from build123d import *

# Parameters (mm, degrees)
SKETCH5_R           = 3.175
BOSS_EXTRUDE3_DEPTH = 88.9
CHAMFER1_SIZE       = 0.77724
BOSS_EXTRUDE4_DEPTH = 4.365625
SKETCH8_OUTSIDE_W   = 358.618
SKETCH8_OUTSIDE_H   = 360.338
SKETCH8_OUTSIDE_R   = 5.55625
CUT_EXTRUDE3_DEPTH  = 94.265625
CUT_EXTRUDE3_TAPER  = 60
CUT_EXTRUDE4_DEPTH  = 0.254
CIRPATTERN1_COUNT   = 3


with BuildPart() as part:
    # Sketch5 → Boss-Extrude3 (new body)
    with BuildSketch(Plane(origin=(46.6328125, 0, 0), x_dir=(0, 0, -1), z_dir=(1, 0, 0))):
        Circle(SKETCH5_R)
    extrude(amount=-BOSS_EXTRUDE3_DEPTH)

    # Chamfer1
    chamfer1_edges = [part.edges().sort_by_distance(p)[0] for p in [
        (46.6328125, 0, 3.175),
    ]]
    chamfer(chamfer1_edges, length=CHAMFER1_SIZE)

    # Sketch6 → Boss-Extrude4 (add)
    with BuildSketch(Plane.ZY.offset(42.2671875)):
        Polygon((5.55625, 3.207902433), (0, 6.415804866), (-5.55625, 3.207902433), (-5.55625, -3.207902433), (0, -6.415804866), (5.55625, -3.207902433), align=None)
    extrude(amount=BOSS_EXTRUDE4_DEPTH)

    # Sketch8 outside → Cut-Extrude3 (cut, through all)
    with BuildSketch(Plane.ZY.offset(46.6328125)):
        Rectangle(SKETCH8_OUTSIDE_W, SKETCH8_OUTSIDE_H)
        Circle(SKETCH8_OUTSIDE_R, mode=Mode.SUBTRACT)
    extrude(amount=-CUT_EXTRUDE3_DEPTH, taper=CUT_EXTRUDE3_TAPER, mode=Mode.SUBTRACT)

    # Sketch12 → Cut-Extrude4 (cut)
    with BuildSketch(Plane.ZY.offset(46.6328125)):
        with BuildLine():
            Line((0.1666875, 4.2783125), (0.1666875, 2.3891875))
            ThreePointArc((0.1666875, 2.3891875), (0, 2.2225), (-0.1666875, 2.3891875))
            Line((-0.1666875, 2.3891875), (-0.1666875, 4.2783125))
            ThreePointArc((-0.1666875, 4.2783125), (0, 4.445), (0.1666875, 4.2783125))
        make_face()
    cut_extrude4 = extrude(amount=-CUT_EXTRUDE4_DEPTH, mode=Mode.SUBTRACT)

    # CirPattern1: Cut-Extrude4 ×3 about axis
    cirpattern1_axis = Axis((0, 0, 0), (1, 0, 0))
    for i in range(1, CIRPATTERN1_COUNT):
        add(cut_extrude4.rotate(cirpattern1_axis, i * 360 / CIRPATTERN1_COUNT), mode=Mode.SUBTRACT)


solid = part.part
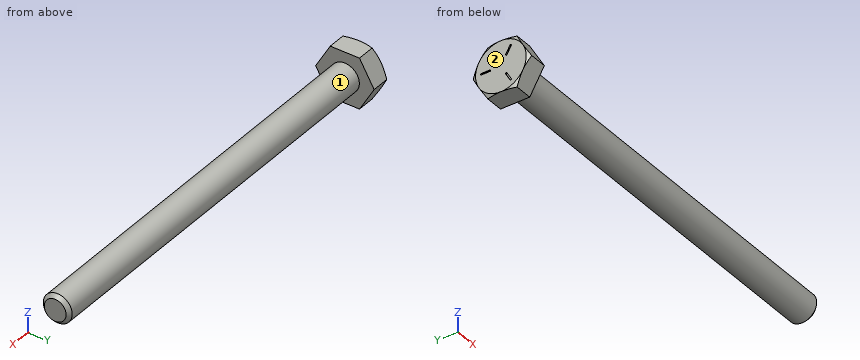
The model under review builds one solid part; all positions refer to its coordinate system, in mm. Face numbers are marked on the shaded views. A direction names the side the tool comes from. Round coordinates to 2 decimals unless told otherwise and drop trailing zeros. Order: outer loops, then holes, each group sorted by start corner. A loop starts at its lowest first (then second) coordinate and runs counter-clockwise, first axis right, second up. Notation, with made-up numbers: (78, 85.5) -> (129, 85.5) arc R19 cw to (129, 91.5) -> close; hole circle Ø10 at (-33.5, -33). An arc over 180 degrees is marked (long way). Return JSON: item names as keys, results as strings.
1. Take a section at A-A (x = 17). Write out the cut boundary in (y, z) (3 decimals), then the cut area to 3 significant figures.
Answer block:
{"outline": "circle Ø6.35 at (0, 0)", "area": "31.7 mm²"}
2. For the marked faces 1 and 2, list the 3-axis set-ups (+Z, -Z, +X, -X, +Y, -Y) from which the entire face can be reached by the end or side of a thin tool; tool diameter is ignored.
Answer block:
{"face 1": "+X", "face 2": "+Z, -Z, -X, +Y, -Y"}
3. For L1, parallel to Y at x = -5.5, z = 0.25; L2, parallel to X at y = -4.5, z = -2.75; L3, parallel to Z at x = -40.5, y = -1.5, list the stretches that pass through material, from the lowest coordinate up. Write a range as [from, to].
Answer block:
{"L1": "y = [-3.17, 3.17]", "L2": "x = [-46.63, -42.27]", "L3": "z = [-2.8, 2.8]"}
4. Insertion check: P1, Ø3, axis at x = -25.5, z = 0.5, coming from the -Y side (3 decimals); P2, Ø3, axis at x = 26, y = 0.5, coming from the +Z side (3 decimals); P3, Ø1, axis at x = -12.5, z = -1, coming from the -Y side. Each pin has a flat end and moves straight along its axis. Give the tip position at first contact, or say it passes through.
Answer block:
{"P1": "stops at y = -3.175", "P2": "stops at z = 3.175", "P3": "stops at y = -3.14"}
